Verification items for the finished model (mm, model axes). A direction names the side the tool comes from. Coordinates: 2 decimals unless noted, no trailing zeros. Write each loop counter-clockwise with the first axis right and the second up, starting at its lowest first coordinate (ties: lowest second). Pieces come first, ordered by that corner, then holes. Notation, with made-up numbers: (-19, 15) -> (-14, 15) arc R27 cw to (-14, 52) -> close; hole circle Ø5 at (-33, 57). An arc over 180 degrees is marked (long way). Answer in a Markdown table with one row per item.
```python
from build123d import *

# Parameters (mm, degrees)
F0_W           = 28
F0_H           = 3
F1_DEPTH       = 50
F2_W           = 1
F2_H           = 2
F3_DEPTH       = 50
F5_D           = 2
F5_CSINK_D     = 3
F5_CSINK_ANGLE = 90
F6_D           = 2
F6_CSINK_D     = 3
F6_CSINK_ANGLE = 90


with BuildPart() as f1:
    # F0 (on Front) → F1 (new body)
    with BuildSketch(Plane.XZ):
        Polygon((0, -3), (0, 0), (-3, 0), (-3, -21), (0, -21), align=None)
        with Locations((14, -1.5)):
            Rectangle(F0_W, F0_H)
        Polygon((31, 0), (28, 0), (28, -3), (28, -21.022089), (31, -21.022089), align=None)
    extrude(amount=F1_DEPTH)

    # F2 (on face) → F3 (cut)
    with BuildSketch(Plane.XZ.offset(50)):
        with Locations((-0.5, -7)):
            Rectangle(F2_W, F2_H)
        with Locations((28.5, -7)):
            Rectangle(F2_W, F2_H)
    extrude(amount=-F3_DEPTH, mode=Mode.SUBTRACT)

    # F5 (through all)
    with Locations(Plane(origin=(0, 0, -3), x_dir=(1, 0, 0), z_dir=(0, 0, -1))):
        with Locations((14, 47)):
            CounterSinkHole(F5_D / 2, F5_CSINK_D / 2, counter_sink_angle=F5_CSINK_ANGLE)

    # F6 (through all)
    with Locations(Plane(origin=(0, 0, -3), x_dir=(1, 0, 0), z_dir=(0, 0, -1))):
        with Locations((14, 3)):
            CounterSinkHole(F6_D / 2, F6_CSINK_D / 2, counter_sink_angle=F6_CSINK_ANGLE)


solid = f1.part
```
1. Mould release check, pull along X, two halves, no side actions. Record for faces 4 (the flat face through (14, -25, -3)), 5 (the flat face through (14, -25, 0)), 6 (the cylindrical face through (13, -3, -1)), 7 (the flat face through (31, -25, -11)): released by +X, released by -X, zero draft, split by the parting line, or undercut.
Geometry says:
| item | result |
|---|---|
| face 4 | undercut |
| face 5 | zero draft |
| face 6 | undercut |
| face 7 | released by +X |
2. Section check D-D, the plane y = -31. Record the boundary of the cut face in (x, z), plus the area to 3 significant figures.
Geometry says:
| item | result |
|---|---|
| outline | (-3, -21) -> (0, -21) -> (0, -8) -> (-1, -8) -> (-1, -6) -> (0, -6) -> (0, -3) -> (28, -3) -> (28, -6) -> (29, -6) -> (29, -8) -> (28, -8) -> (28, -21.02) -> (31, -21.02) -> (31, 0) -> (-3, 0) -> close |
| area | 206 mm^2 |
3. Depth check by flat-ended pin: P1, Ø8.5, axis at x = 13, y = -21.5, coming from the -Z side; P2, Ø4, axis at x = 25, z = -13.5, coming from the +Y side; P3, Ø1.1, axis at x = -0.5, y = -37, coming from the -Z side; P4, Ø2.5, axis at x = 14, y = -3, coming from the -Z side. Enter the tip coordinate at first touch or a pass-through.
Geometry says:
| item | result |
|---|---|
| P1 | z = -3 |
| P2 | through |
| P3 | z = -21 |
| P4 | z = -2.75 |
4. Section check A-A, the plane x = 14. Record the boundary of the cut face in (y, z).
Geometry says:
| item | result |
|---|---|
| outline | (-50, -3) -> (-48.5, -3) -> (-48, -2.5) -> (-48, 0) -> (-50, 0) -> close; (-46, -2.5) -> (-45.5, -3) -> (-4.5, -3) -> (-4, -2.5) -> (-4, 0) -> (-46, 0) -> close; (-2, -2.5) -> (-1.5, -3) -> (0, -3) -> (0, 0) -> (-2, 0) -> close |
5. Section check B-B, the plane y = -47. Record the boundary of the cut face in (x, z), plus the area to 3 significant figures.
Geometry says:
| item | result |
|---|---|
| outline | (-3, -21) -> (0, -21) -> (0, -8) -> (-1, -8) -> (-1, -6) -> (0, -6) -> (0, -3) -> (12.5, -3) -> (13, -2.5) -> (13, 0) -> (-3, 0) -> close; (15, -2.5) -> (15.5, -3) -> (28, -3) -> (28, -6) -> (29, -6) -> (29, -8) -> (28, -8) -> (28, -21.02) -> (31, -21.02) -> (31, 0) -> (15, 0) -> close |
| area | 200 mm^2 |
6. Thickness scan on line 1 (Y direction, x = 14, z = -1.55); line 2 (X direction, y = -39.5, z = -5); line 3 (X direction, y = -47, z = -1.25). Record the ranges inside material, lowest first. Write a range as from..to.
Geometry says:
| item | result |
|---|---|
| line 1 | -50..-48, -46..-4, -2..0 |
| line 2 | -3..0, 28..31 |
| line 3 | -3..13, 15..31 |
7. Tool access check on faces 1 (the flat face through (0, -25, -5)), 2 (the flat face through (-0.5, -25.4, -8)), 3 (the flat face through (13.9, 0, -2.7)). Record the directions out of +Z, -Z, +X, -X, +Y, -Y that give a thin tool (end or side, any length) a straight path to the whole face; none if there is none.
Geometry says:
| item | result |
|---|---|
| face 1 | -Z, +Y, -Y |
| face 2 | +Y, -Y |
| face 3 | +Z, -Z, +X, -X, +Y |
8. Section check C-C, the plane z = -11.75. Record the boundary of the cut face in (x, y).
Geometry says:
| item | result |
|---|---|
| outline | (-3, -50) -> (0, -50) -> (0, 0) -> (-3, 0) -> close; (28, -50) -> (31, -50) -> (31, 0) -> (28, 0) -> close |
